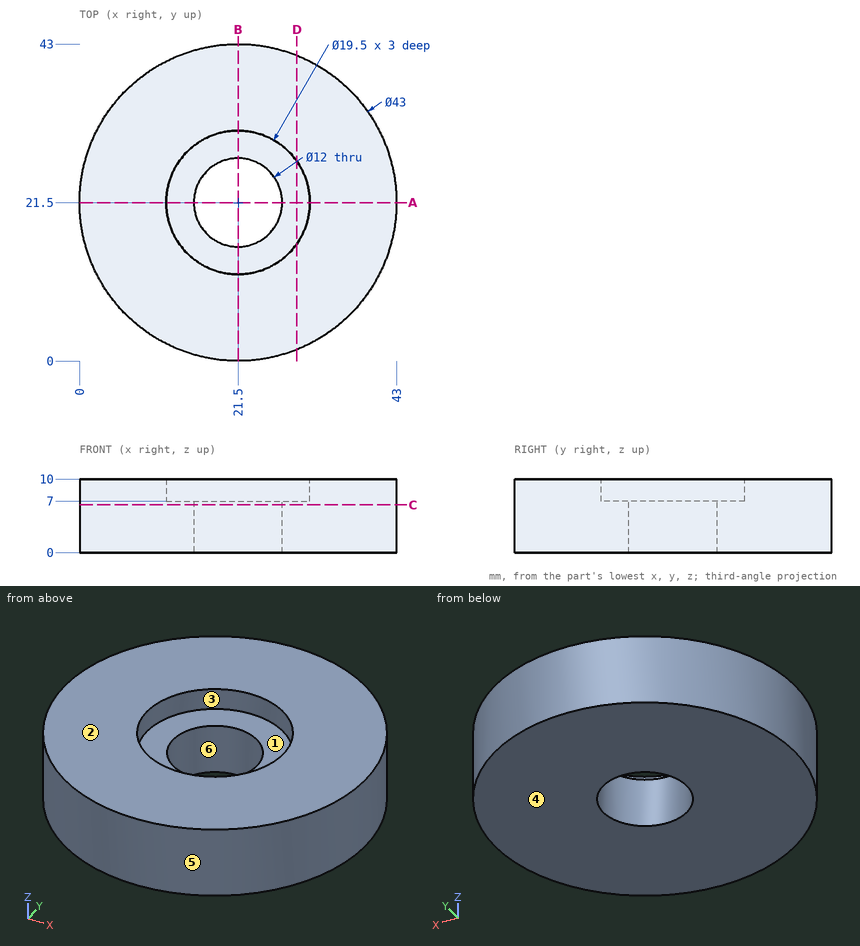
Can you work these out from the drawing? Everything is in mm from the part's minimum corner. A direction names the side the tool comes from. Round coordinates to 2 decimals unless told otherwise and drop trailing zeros. Loops run counter-clockwise (first coordinate to the right, second up) from the corner with the lowest first, then second, coordinate; pieces in that order, holes last. Notation, with made-up numbers: (28.25, 17) - (63.25, 17) arc R18 ccw to (63.25, 41) - close; hole circle Ø2 at (14.25, -5.75). An arc over 180 degrees is marked (long way). Answer in a Markdown table with one row per item. Add a question column.
Q1. I want a section at A-A on y = 21.5. List the corners of the cut face in (x, z) for me, and give its area (4 significant figures).
Q2. I need wall thicknesses on L1, parallel to Y at x = 21.5, z = 2.25; L2, parallel to Y at x = 21.5, z = 8.9; L3, parallel to X at y = 20.5, z = 8.5. Which ranges of each line are inside material? Lowest first, please.
Q3. We'd pull the mould along X, two halves only. Please class the marked faces 3, 4, 5 and 6: pulls with the +X half, pulls with the -X half, needs draft (parallel to the pull), parting line crosses it, or undercut.
Q4. I want a section at D-D on x = 29.5. List the corners of the cut face in (y, z) for me, and give its area (3 significant figures).
Q5. I want a section at C-C on z = 6.5. List the corners of the cut face in (x, y) for me.
Q6. Which directions (+Z, -Z, +X, -X, +Y, -Y) give clear straight access to the entire face, cutting with the end or side of a thin tool? Please do the marked faces 1 and 2.
Q7. For pin 1 Ø1.5 at (x, z) = (26, 6) entering from +Y; pin 2 Ø19 at (x, y) = (21.5, 21.5) entering from +Z; pin 3 Ø1.5 at (x, z) = (22, 2.5) entering from -Y, each with a flat end and sliding along its axis, tell me the tip position at first contact or that it passes through.
A:
| question | item | result |
|---|---|---|
| 1 | outline | (0, 0) - (15.5, 0) - (15.5, 7) - (11.75, 7) - (11.75, 10) - (0, 10) - close; (27.5, 0) - (43, 0) - (43, 10) - (31.25, 10) - (31.25, 7) - (27.5, 7) - close |
| 1 | area | 287.5 mm^2 |
| 2 | L1 | 0 to 15.5, 27.5 to 43 |
| 2 | L2 | 0 to 11.75, 31.25 to 43 |
| 2 | L3 | 0.02 to 11.8, 31.2 to 42.98 |
| 3 | face 3 | undercut |
| 3 | face 4 | needs draft |
| 3 | face 5 | parting line crosses it |
| 3 | face 6 | undercut |
| 4 | outline | (1.54, 0) - (41.46, 0) - (41.46, 10) - (27.07, 10) - (27.07, 7) - (15.93, 7) - (15.93, 10) - (1.54, 10) - close |
| 4 | area | 366 mm^2 |
| 5 | outline | circle Ø43 at (21.5, 21.5); hole circle Ø12 at (21.5, 21.5) |
| 6 | face 1 | +Z |
| 6 | face 2 | +Z, +X, -X, +Y, -Y |
| 7 | pin 1 | y = 42.67 |
| 7 | pin 2 | z = 7 |
| 7 | pin 3 | y = 0 |
